Build history of the part. All positions in model axes, mm. Face numbers are marked on the shaded views. Round coordinates to 2 decimals unless told otherwise and drop trailing zeros. Order: outer loops, then holes, each group sorted by start corner. A loop starts at its lowest first (then second) coordinate and runs counter-clockwise, first axis right, second up. Notation, with made-up numbers: M -5.75,-38.75 L 1.25,-38.75 A30 cw 1.25,-11.75 Z; hole C -28,86.25 d9. An arc over 180 degrees is marked long. One line per item, written item: value. Start each with the question number.
Item 1: Band-saw the part on B-B, the plane y = -5. Write the cut outline in (x, z), then the cut area to 3 significant figures.
Item 2: Band-saw the part on D-D, the plane y = -30. Write the cut outline in (x, z), then the cut area to 3 significant figures.
Item 3: Pin check, flat tips, straight feed: pin 1 (3 mm diameter, centred on x = -43.5, y = -12.5, fed in from -Z); pin 2 (0.9 mm diameter, centred on x = -40.5, y = -12, fed in from -Z); pin 3 (1 mm diameter, centred on y = -7.5, z = 12, fed in from -X). Stop position of each tip, or through.
Item 4: Two-plate mould, pull along Y, no slides. Class the marked faces 1, 2, 3 and 4: +Y half, -Y half, draft (parallel to the pull), parting line (faces both ways), or undercut.
Item 5: Band-saw the part on C-C, the plane z = 21.5. Write the cut outline in (x, y), then the cut area to 3 significant figures.
Item 6: Probe L1, parallel to Z at x = -43.5, y = 2; L2, parallel to X at y = -2.85, z = -42; L3, parallel to Y at x = -42, z = 28.5. List the from-to ranges inside material, lowest first.
Item 7: Band-saw the part on A-A, the plane z = -30. Write the cut outline in (x, y).
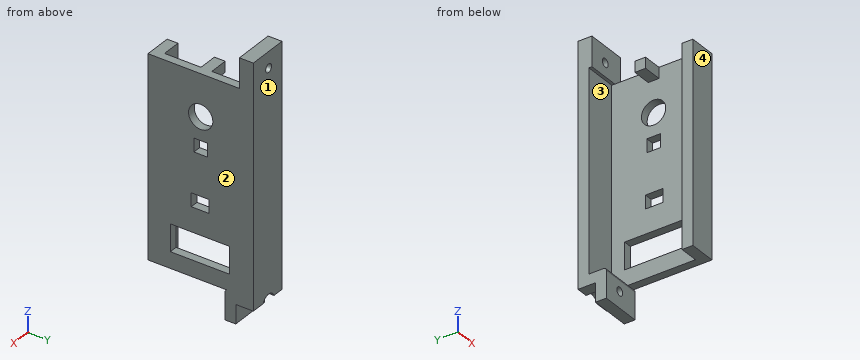
```python
from build123d import *

# Parameters (mm, degrees)
EXTRUDE_START       = -12
EXTRUDE_1_DEPTH     = 12
SKETCH_2_R          = 4.5
EXTRUDE_2_DEPTH     = 3
SKETCH_3_W          = 74
SKETCH_3_H          = 4
SKETCH_3_W_2        = 4
EXTRUDE_3_DEPTH     = 7
SKETCH_4_W          = 5
SKETCH_4_H          = 6.5
SKETCH_4_H_2        = 5
SKETCH_4_W_2        = 10
SKETCH_4_H_3        = 22
CUT_EXTRUDE_1_DEPTH = 7
SKETCH_5_R          = 1.55
CUT_EXTRUDE_2_DEPTH = 7
SKETCH_6_R          = 3
CUT_EXTRUDE_4_DEPTH = 7
SKETCH_8_W          = 123.006467786
SKETCH_8_H          = 80.173858468
CUT_EXTRUDE_6_DEPTH = 15
SKETCH_11_R         = 1.55
EXTRUDE_5_DEPTH     = 5.15
CUT_EXTRUDE_8_REACH = 107.579
SKETCH_12_W         = 15.113452747
SKETCH_12_H         = 5.35


# Read off the part's stored shape, not the designer's step: 填料-伸長1
with BuildPart() as part:
    # 填料-伸長1 outline → 填料-伸長1 (new body)
    with BuildSketch(Plane.ZY.offset(65.537274581).offset(EXTRUDE_START)):
        with BuildLine():
            Line((41, 0.007142857), (41, 6.507142857))
            Line((41, 6.507142857), (-41, 6.507142857))
            Line((-41, 6.507142857), (-41, 0.007142857))
            Line((-41, 0.007142857), (-48, 0.007142857))
            Line((-48, 0.007142857), (-48, -3.992857143))
            Line((-48, -3.992857143), (-38, -3.992857143))
            ThreePointArc((-38, -3.992857143), (-37.292893219, -3.699963924), (-37, -2.992857143))
            Line((-37, -2.992857143), (-37, 2.507142857))
            Line((-37, 2.507142857), (37, 2.507142857))
            Line((37, 2.507142857), (37, -2.992857143))
            ThreePointArc((37, -2.992857143), (37.292893219, -3.699963924), (38, -3.992857143))
            Line((38, -3.992857143), (48, -3.992857143))
            Line((48, -3.992857143), (48, 0.007142857))
            Line((48, 0.007142857), (41, 0.007142857))
        make_face()
    extrude(amount=EXTRUDE_1_DEPTH)

    # 草圖2 → 填料-伸長2 (add)
    # profile 1 of 2: a face of its own
    with BuildSketch(Plane.ZY.offset(65.537274581)):
        Polygon((37, 2.507142857), (-37, 2.507142857), (-37, -2.992857143), (-37, -32.492857143), (37, -32.492857143), (37, -2.992857143), align=None)
        with Locations((21.5, -12.992857143)):
            Circle(SKETCH_2_R, mode=Mode.SUBTRACT)
    # profile 2 of 2: a face of its own
    with BuildSketch(Plane.ZY.offset(65.537274581)):
        with BuildLine():
            Line((41, 0.007142857), (41, 6.507142857))
            Line((41, 6.507142857), (-41, 6.507142857))
            Line((-41, 6.507142857), (-41, 0.007142857))
            Line((-41, 0.007142857), (-48, 0.007142857))
            Line((-48, 0.007142857), (-48, -3.992857143))
            Line((-48, -3.992857143), (-38, -3.992857143))
            ThreePointArc((-38, -3.992857143), (-37.292893219, -3.699963924), (-37, -2.992857143))
            Line((-37, -2.992857143), (-37, 2.507142857))
            Line((-37, 2.507142857), (37, 2.507142857))
            Line((37, 2.507142857), (37, -2.992857143))
            ThreePointArc((37, -2.992857143), (37.292893219, -3.699963924), (38, -3.992857143))
            Line((38, -3.992857143), (48, -3.992857143))
            Line((48, -3.992857143), (48, 0.007142857))
            Line((48, 0.007142857), (41, 0.007142857))
        make_face()
    extrude(amount=EXTRUDE_2_DEPTH)

    # 草圖3 → 填料-伸長3 (add)
    with BuildSketch(Plane(origin=(-65.537274581, 0, 0), x_dir=(0, 0, -1), z_dir=(1, 0, 0))):
        with Locations((0, -30.492857143)):
            Rectangle(SKETCH_3_W, SKETCH_3_H)
        with Locations((-35, -12.992857143)):
            Rectangle(SKETCH_3_W_2, SKETCH_3_H)
    extrude(amount=EXTRUDE_3_DEPTH)

    # 草圖4 → 除料-伸長1 (cut)
    with BuildSketch(Plane.ZY.offset(68.537274581)):
        with Locations((-9.5, -13.242857143)):
            Rectangle(SKETCH_4_W, SKETCH_4_H)
        with Locations((10.5, -12.992857143)):
            Rectangle(SKETCH_4_W, SKETCH_4_H_2)
        with Locations((-26, -13.242857143)):
            Rectangle(SKETCH_4_W_2, SKETCH_4_H_3)
    extrude(amount=-CUT_EXTRUDE_1_DEPTH, mode=Mode.SUBTRACT)

    # 草圖5 → 除料-伸長2 (cut)
    with BuildSketch(Plane(origin=(0, 0.007142857, 0), x_dir=(1, 0, 0), z_dir=(0, 1, 0))):
        with Locations(Location((-60.537274581, -42, 0), (0, 0, 40.17776954))):
            Circle(SKETCH_5_R)
        with Locations(Location((-60.537274581, 42, 0), (0, 0, 220.17776954))):
            Circle(SKETCH_5_R)
    extrude(amount=-CUT_EXTRUDE_2_DEPTH, mode=Mode.SUBTRACT)

    # 草圖6 → 除料-伸長4 (cut)
    with BuildSketch(Plane(origin=(0, 0.007142857, 0), x_dir=(1, 0, 0), z_dir=(0, 1, 0))):
        with Locations((-60.537274581, -42)):
            Circle(SKETCH_6_R)
        with Locations((-60.537274581, 42)):
            Circle(SKETCH_6_R)
    extrude(amount=CUT_EXTRUDE_4_DEPTH, mode=Mode.SUBTRACT)

    # 鏡射2: part across plane


with BuildPart() as part_1:
    add(part.part)
    add(part.part.mirror(Plane(origin=(-53.537274581, 0, 0), x_dir=(0, 0, 1), z_dir=(1, 0, 0))))

    # 草圖8 → 除料-伸長6 (cut)
    with BuildSketch(Plane(origin=(-53.537274581, 0, 0), x_dir=(0, 0, -1), z_dir=(1, 0, 0))):
        with Locations((-0.366090678, -13.819923092)):
            Rectangle(SKETCH_8_W, SKETCH_8_H)
    extrude(amount=-CUT_EXTRUDE_6_DEPTH, mode=Mode.SUBTRACT)

    # 草圖11 → 填料-伸長5 (add)
    with BuildSketch(Plane(origin=(0, 1.357142857, 0), x_dir=(-1, 0, 0), z_dir=(0, -1, 0))):
        with BuildLine():
            Line((53.537274581, -48), (53.537274581, -41))
            Line((53.537274581, -41), (49.365701705, -41))
            ThreePointArc((49.365701705, -41), (46.537274581, -39), (43.708847456, -41))
            Line((43.708847456, -41), (38.537274581, -41))
            Line((38.537274581, -41), (38.537274581, -48))
            Line((38.537274581, -48), (53.537274581, -48))
        make_face()
        with Locations(Location((46.537274581, -42, 0), (0, 0, 270))):
            Circle(SKETCH_11_R, mode=Mode.SUBTRACT)
    extrude(amount=-EXTRUDE_5_DEPTH)

    # 草圖12 → 除料-伸長8 (cut, up to next)
    with BuildSketch(Plane.XY.offset(37), mode=Mode.PRIVATE) as cut_extrude_8_sk1:
        with Locations((-46.094000955, -1.317857143)):
            Rectangle(SKETCH_12_W, SKETCH_12_H)
    cut_extrude_8_tool1 = extrude(cut_extrude_8_sk1.sketch, amount=CUT_EXTRUDE_8_REACH, mode=Mode.PRIVATE) & part_1.part
    add(cut_extrude_8_tool1.solids().sort_by_distance((-46.094001, -1.317857, 37))[0], mode=Mode.SUBTRACT)


solid = part_1.part
```
Output:
1. outline: M -41.54,-37 L -38.54,-37 L -38.54,-31 L -41.54,-31 Z; M -41.54,-21 L -38.54,-21 L -38.54,37 L -41.54,37 Z
1. area: 192 mm²
2. outline: M -48.54,-37 L -38.54,-37 L -38.54,37 L -48.54,37 Z
2. area: 740 mm²
3. pin 1: stops at z = 33
3. pin 2: stops at z = -37
3. pin 3: stops at x = -41.54
4. face 1: +Y half
4. face 2: draft
4. face 3: undercut
4. face 4: -Y half
5. outline: M -53.54,2.51 L -41.54,2.51 L -41.54,-8.49 L -38.54,-8.49 L -38.54,6.51 L -53.54,6.51 Z; M -48.54,-32.49 L -38.54,-32.49 L -38.54,-17.49 L -41.54,-17.49 L -41.54,-28.49 L -48.54,-28.49 Z
5. area: 166 mm²
6. L1: z = -41 to -37, 37 to 48
6. L2: x = -53.54 to -48.09, -44.99 to -38.54
6. L3: y = -32.49 to -28.49, 2.51 to 6.51
7. outline: M -53.54,2.51 L -41.54,2.51 L -41.54,-2.24 L -38.54,-2.24 L -38.54,6.51 L -53.54,6.51 Z; M -48.54,-32.49 L -38.54,-32.49 L -38.54,-24.24 L -41.54,-24.24 L -41.54,-28.49 L -48.54,-28.49 Z
